Geometry: final body of the model. Coordinates: model frame, mm. A direction names the side the tool comes from. Give positions to 0.01 mm unless a question says otherwise; leave off trailing zeros. Write each loop counter-clockwise with the first axis right and the second up, starting at its lowest first coordinate (ties: lowest second). Pieces come first, ordered by that corner, then holes. Notation, with made-up numbers: (-30, 21.5) -> (-13, 21.5) arc R21 cw to (-13, 27.5) -> close; hole circle Ø1 at (-19, -21). An arc over 180 degrees is marked (long way). Answer as a JSON object with one key per item and string values. Group by question number.
(1) Draft query along X for faces 1 (the face through (-10.94, 61.34, 49.3)), 2 (the face through (23.873, 183.911, 10.14)), 3 (the face through (51, -10, -10)). Return one class per face: +X half, -X half, draft (parallel to the pull), parting line (faces both ways), or undercut.
(2) Set-up query: faces 4 (the face through (110, 16, 90)), 5 (the face through (48, 101, 0)), 6 (the face through (-10, -10, 49)), 7 (the face through (110, -10, 51)), 8 (the face through (54, 30, 20)). Return all of +Z, -Z, +X, -X, +Y, -Y with unobstructed straight access to the full face (end or side cutting, diameter ignored); none if empty.
(3) Section query C-C on y = 92. Output: boundary loops of the cut face in (x, z), plus the area to 3 significant figures.
(4) Contact query for flat-ended pins moving along their axis: pin 1 Ø12 at (x, y) = (-7.28, 121.51) entering from +Z; pin 2 Ø1 at (y, z) = (163, 96.5) entering from -X; pin 3 Ø12 at (x, y) = (19, 46) entering from -Z; pin 4 Ø18 at (x, y) = (61, 26) entering from +Z. Output: stop coordinate, or through.
(5) Section query B-B on x = 31.5. Output: boundary loops of the cut face in (y, z), plus the area to 3 significant figures.
(6) Material intervals for probe 1 along Z at (x, y) = (80.5, 39.5); probe 2 along Y at (x, z) = (88, 62); probe 3 along Z at (x, y) = (0, 72.5), sorted ascending.
(7) Section query D-D on y = 126.5. Output: boundary loops of the cut face in (x, z), plus the area to 3 significant figures.
(8) Section query A-A on z = 60. Output: boundary loops of the cut face in (x, y).
Autodesk Inventor part; units mm, degrees
ref_plane "YZ Plane" through (0, 0, 0) normal (1, 0, 0) x (0, 1, 0)
ref_plane "XZ Plane" through (0, 0, 0) normal (0, 1, 0) x (-1, 0, 0)
ref_plane "XY Plane" through (0, 0, 0) normal (0, 0, 1) x (1, 0, 0)
sketch "Sketch1" plane through (0, 0, 0) normal (0, 0, 1) x (1, 0, 0)
  line L0 (0, 0) -> (100, 0)
  line L1 (0, 200) -> (150, 200)
  line L2 (150, 200) -> (150, 80)
  line L3 (150, 80) -> (100, 0)
  line L4 (0, 200) -> (-23.9414, 134.2215)
  line L5 (0, 200) -> (70, 200) construction
  line L6 (-23.9414, 134.2215) -> (0, 0)
extrude "Extrusion1" add sketch "Sketch1" along normal blind 120
fillet "Fillet1" radius 50 1 edges at (-23.9414, 134.2215, 60)
sketch "Sketch3" plane through (0, 0, 120) normal (0, 0, 1) x (1, 0, 0)
  line L0 (0, 200) -> (-19.341, 146.861)
  circle A0 centre (14.3344, 180.9074) radius 10
  line L1 (14.3344, 180.9074) -> (10.9142, 171.5105)
  line L2 (14.3344, 180.9074) -> (133.919, 180.9074) construction
  circle A1 centre (3.6348, 151.5105) radius 10
  circle A2 centre (-7.2843, 121.5105) radius 10
  dimension "d9" = 20
  dimension "d10" = 20
  dimension "d12" = 20
  dimension "d13" = 20
  dimension "d14" = 30
  dimension "d15" = 20
extrude "Extrusion2" cut sketch "Sketch3" against normal blind 120
sketch "Sketch4" plane through (0, 0, 0) normal (1, 0, 0) x (0, 1, 0)
  line L0 (0, 0) -> (200, 0)
  line L1 (200, 100) -> (0, 100)
  line L2 (200, 20) -> (0, 80) construction
  line L3 (0, 20) -> (200, 80) construction
  line L4 (200, 0) -> (200, 20)
  line L5 (200, 80) -> (200, 100)
  line L6 (0, 100) -> (0, 80)
  line L7 (0, 20) -> (0, 0)
  line L8 (60, 50) -> (60, 20)
  line L9 (60, 50) -> (60, 80)
  line L10 (75, 80) -> (75, 20)
  line L11 (200, 20) -> (75, 20)
  line L12 (60, 20) -> (0, 20)
  line L13 (0, 80) -> (60, 80)
  line L14 (75, 80) -> (200, 80)
  point P0 (100, 50)
extrude "Extrusion3" cut sketch "Sketch4" along normal mid plane 240 keep common part
sketch "Sketch5" plane through (0, 0, 0) normal (0, 1, 0) x (-1, 0, 0)
  line L0 (10, 110) -> (-110, 110)
  line L1 (-110, 110) -> (-110, -10)
  line L2 (-110, -10) -> (10, -10)
  line L3 (10, -10) -> (10, 110)
  line L4 (10, 110) -> (-110, -10) construction
  line L5 (-110, 110) -> (10, -10) construction
  point P0 (0, 0)
  dimension "d28" = 120
  dimension "d29" = 120
extrude "Extrusion4" add sketch "Sketch5" against normal blind 20
properties part number "BADAN 3"
Answer list:
{
 "1": {"face 1": "-X half", "face 2": "undercut", "face 3": "draft"},
 "2": {"face 4": "+Z, -Z, +X", "face 5": "-Z, +X, -X, +Y", "face 6": "+Z, -Z, -X, -Y", "face 7": "+Z, -Z, +X, -Y", "face 8": "+X, -X"},
 "3": {"outline": "(-16.41, 0) -> (120, 0) -> (120, 20) -> (-16.41, 20) -> close; (-16.41, 80) -> (120, 80) -> (120, 100) -> (-16.41, 100) -> close", "area": "5,460 mm2"},
 "4": {"pin 1": "through", "pin 2": "x = -13.65", "pin 3": "z = 0", "pin 4": "z = 100"},
 "5": {"outline": "(-20, -10) -> (0, -10) -> (0, 0) -> (200, 0) -> (200, 20) -> (75, 20) -> (75, 80) -> (200, 80) -> (200, 100) -> (0, 100) -> (0, 110) -> (-20, 110) -> close; hole (0, 20) -> (60, 20) -> (60, 80) -> (0, 80) -> close", "area": "11,300 mm2"},
 "6": {"probe 1": "0 to 20, 80 to 100", "probe 2": "-20 to 0, 60 to 75", "probe 3": "0 to 100"},
 "7": {"outline": "(-22.25, 0) -> (-15.95, 0) -> (-15.95, 20) -> (-22.25, 20) -> close; (-22.25, 80) -> (-15.95, 80) -> (-15.95, 100) -> (-22.25, 100) -> close; (1.38, 0) -> (120, 0) -> (120, 20) -> (1.38, 20) -> close; (1.38, 80) -> (120, 80) -> (120, 100) -> (1.38, 100) -> close", "area": "5,000 mm2"},
 "8": {"outline": "(-13.38, 75) -> (-10.7, 60) -> (120, 60) -> (120, 75) -> close; (-10, -20) -> (110, -20) -> (110, 0) -> (-10, 0) -> close"}
}
